Source: three-view drawing plus pictorial views. Frame: mm from the lowest corner of the part. A direction names the side the tool comes from. Give positions to 0.01 mm unless a question says otherwise; leave off trailing zeros. Write each loop counter-clockwise with the first axis right and the second up, starting at its lowest first coordinate (ties: lowest second). Pieces come first, ordered by that corner, then holes. Notation, with made-up numbers: M -13,38 L 31,38 A30 cw 31,64 Z; hole C 8.5,-1.75 d1. An arc over 180 degrees is marked long. Return JSON: item names as keys, results as strings.
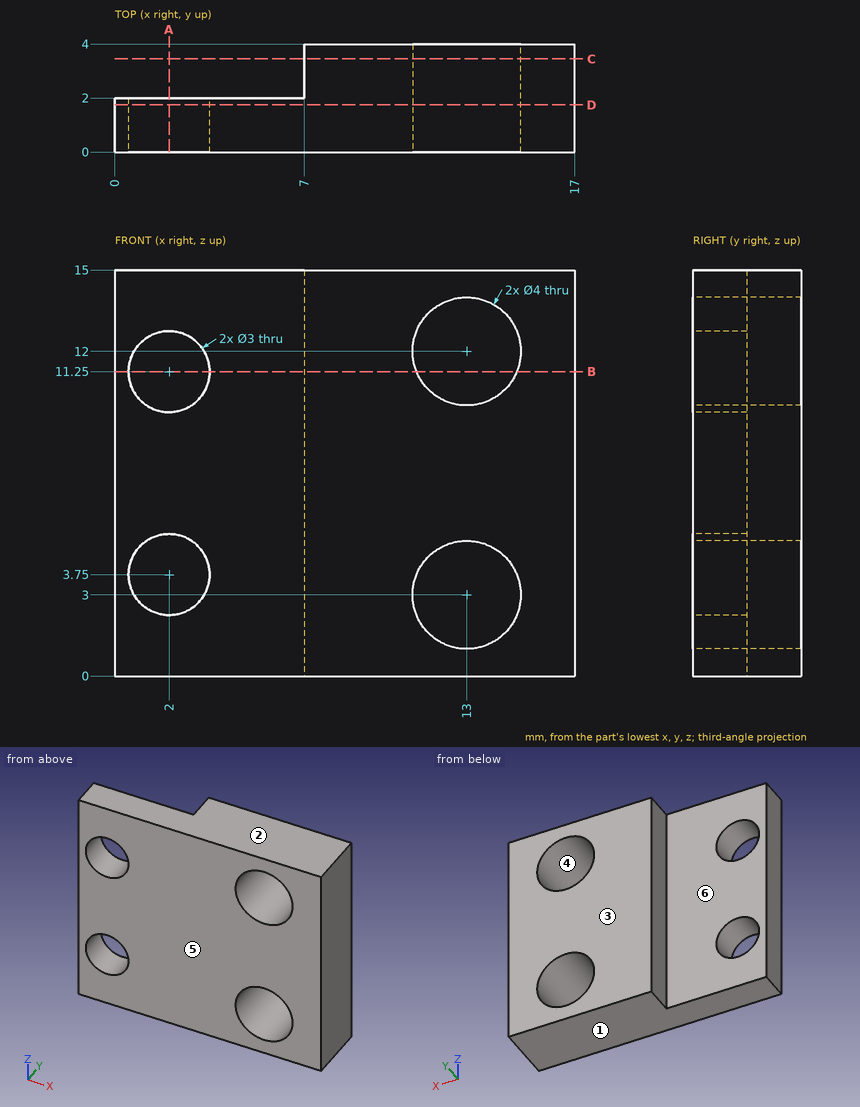
1) Contact query for flat-ended pins moving along their axis: pin 1 Ø6.5 at (x, z) = (13, 3) entering from +Y; pin 2 Ø2 at (x, z) = (5, 6.5) entering from +Y; pin 3 Ø3.5 at (x, z) = (13, 12) entering from -Y; pin 4 Ø0.6 at (y, z) = (3.5, 10.5) entering from -X. Output: stop coordinate, or through.
Numbers:
{"pin 1": "stops at y = 4", "pin 2": "stops at y = 2", "pin 3": "passes through", "pin 4": "stops at x = 7"}
2) Cut plane A-A, the plane x = 2. Return the cut outline in (y, z), then the cut area to 3 significant figures.
Numbers:
{"outline": "M 0,0 L 2,0 L 2,2.25 L 0,2.25 Z; M 0,5.25 L 2,5.25 L 2,9.75 L 0,9.75 Z; M 0,12.75 L 2,12.75 L 2,15 L 0,15 Z", "area": "18.0 mm²"}
3) Line query: line 1 (Z direction, x = 2, y = 1.5); line 2 (Z direction, x = 13, y = 1); line 3 (X direction, y = 0.5, z = 11.5). Output: solid intervals per line, ascending. Write a range as [from, to].
Numbers:
{"line 1": "z = [0, 2.25], [5.25, 9.75], [12.75, 15]", "line 2": "z = [0, 1], [5, 10], [14, 15]", "line 3": "x = [0, 0.52], [3.48, 11.06], [14.94, 17]"}
4) Cut plane D-D, the plane y = 1.75. Return the cut outline in (x, z), then the cut area to 3 significant figures.
Numbers:
{"outline": "M 0,0 L 17,0 L 17,15 L 0,15 Z; hole C 2,3.75 d3; hole C 2,11.25 d3; hole C 13,3 d4; hole C 13,12 d4", "area": "216 mm²"}
5) Set-up query: the marked faces 5 and 6. Return all of +Z, -Z, +X, -X, +Y, -Y with unobstructed straight access to the full face (end or side cutting, diameter ignored); none if empty.
Numbers:
{"face 5": "+Z, -Z, +X, -X, -Y", "face 6": "+Z, -Z, -X, +Y"}
6) Cut plane B-B, the plane z = 11.25. Return the cut outline in (x, y).
Numbers:
{"outline": "M 0,0 L 0.5,0 L 0.5,2 L 0,2 Z; M 3.5,0 L 11.15,0 L 11.15,4 L 7,4 L 7,2 L 3.5,2 Z; M 14.85,0 L 17,0 L 17,4 L 14.85,4 Z"}
7) Cut plane C-C, the plane y = 3.45. Return the cut outline in (x, z), then the cut area to 3 significant figures.
Numbers:
{"outline": "M 7,0 L 17,0 L 17,15 L 7,15 Z; hole C 13,3 d4; hole C 13,12 d4", "area": "125 mm²"}
8) Draft query along Z for the marked faces 1, 2, 3 and 4. Return one class per face: released by +Z, released by -Z, zero draft, split by the parting line, or undercut.
Numbers:
{"face 1": "released by -Z", "face 2": "released by +Z", "face 3": "zero draft", "face 4": "undercut"}
